```python
from build123d import *

# Parameters (mm, degrees)
SKETCH_R        = 35
SKETCH_R_2      = 32.5
PAD_DEPTH       = 2
SKETCH001_R     = 51
SKETCH001_R_2   = 32.5
PAD001_DEPTH    = 3
SKETCH002_R     = 41
SKETCH002_R_2   = 37.5
PAD002_DEPTH    = 10
SKETCH003_R     = 1.6
POCKET_DEPTH    = 5.001
CHAMFER_SIZE    = 0.5
CHAMFER001_SIZE = 1


with BuildPart() as part:
    # Sketch → Pad (new body)
    with BuildSketch(Plane.XY):
        Circle(SKETCH_R)
        Circle(SKETCH_R_2, mode=Mode.SUBTRACT)
    extrude(amount=PAD_DEPTH)

    # Sketch001 (on Face4 of Pad) → Pad001 (join)
    with BuildSketch(Plane.XY.offset(2)):
        Circle(SKETCH001_R)
        Circle(SKETCH001_R_2, mode=Mode.SUBTRACT)
    extrude(amount=PAD001_DEPTH)

    # Sketch002 (on Face7 of Pad001) → Pad002 (join)
    with BuildSketch(Plane.XY.offset(5)):
        Circle(SKETCH002_R)
        Circle(SKETCH002_R_2, mode=Mode.SUBTRACT)
    extrude(amount=PAD002_DEPTH)

    # Sketch003 (on Face7 of Pad002) → Pocket (cut, through all)
    with BuildSketch(Plane.XY.offset(5)):
        with Locations((-23, 39.837169)):
            Circle(SKETCH003_R)
        with Locations((23, 39.837169)):
            Circle(SKETCH003_R)
        with Locations((46, 0)):
            Circle(SKETCH003_R)
        with Locations((23, -39.837169)):
            Circle(SKETCH003_R)
        with Locations((-23, -39.837169)):
            Circle(SKETCH003_R)
        with Locations((-46, 0)):
            Circle(SKETCH003_R)
    extrude(amount=-POCKET_DEPTH, mode=Mode.SUBTRACT)

    # Chamfer
    chamfer_edges = [part.edges().sort_by_distance(p)[0] for p in [
        (-35, 0, 0),
    ]]
    chamfer(chamfer_edges, length=CHAMFER_SIZE)

    # Chamfer001
    chamfer001_edges = [part.edges().sort_by_distance(p)[0] for p in [
        (-37.5, 0, 15),
    ]]
    chamfer(chamfer001_edges, length=CHAMFER001_SIZE)


solid = part.part
```
For this review, take the finished solid that the model builds, in its own axes (mm). A direction names the side the tool comes from. Give positions to 0.01 mm unless a question says otherwise; leave off trailing zeros. Write each loop counter-clockwise with the first axis right and the second up, starting at its lowest first coordinate (ties: lowest second). Pieces come first, ordered by that corner, then holes.
Item 1: The part is to be moulded in two halves that separate along X. For faces 1 (the face through (-22.9, 34.2, 5)), 2 (the face through (22.792, 41.424, 3.521)), 3 (the face through (-11.056, -49.787, 3.479)), say which applies: +X half, -X half, draft (parallel to the pull), parting line (faces both ways), or undercut.
Item 2: Insertion check: P1, Ø3.5, axis at x = 46, y = 0, coming from the -Z side; P2, Ø10, axis at x = 38, y = -28, coming from the +Z side; P3, Ø3, axis at x = -7, z = 9, coming from the +Y side. Each pin has a flat end and moves straight along its axis. Give the tip position at first contact, or say it passes through.
Item 3: Machinability: for faces 4 (the face through (-4.88, 37.18, 9.44)), 5 (the face through (-47.18, 1.08, 3.52)), 6 (the face through (-28, -21, 1)), which of the approach directions +Z, -Z, +X, -X, +Y, -Y give a long, thin tool a straight path to every point of the face, cutting with its end or side? Answer none if there is none.
Item 4: Take a section at C-C (z = 12.25). Give the boundary of the cut face in (x, y), and give its area (3 significant figures).
Item 5: Take a section at A-A (y = 0). Give the number of separate pieces and of enclosed holes in the cut face, and give its area (3 significant figures).
Item 6: Take a section at B-B (x = 0). Give the boundary of the cut face in (y, z), and give its area (3 significant figures).
Item 7: Wall thickness on probe 1 along Y at (x, z) = (0, 2.45); probe 2 along Z at (x, y) = (-30.5, 38); probe 3 along Y at (x, z) = (0, 12): over which ranges is each line inside the solid? List them lowest first.
Established:
1. face 1: draft
1. face 2: undercut
1. face 3: parting line
2. P1: stops at z = 2
2. P2: stops at z = 5
2. P3: stops at y = 40.63
3. face 4: +Z
3. face 5: +Z, -Z
3. face 6: -Z
4. outline: circle Ø82 at (0, 0); hole circle Ø75 at (0, 0)
4. area: 863 mm2
5. separate pieces: 4
5. enclosed holes: 0
5. area: 171 mm2
6. outline: (-51, 2) - (-35, 2) - (-35, 0.5) - (-34.5, 0) - (-32.5, 0) - (-32.5, 5) - (-37.5, 5) - (-37.5, 14) - (-38.5, 15) - (-41, 15) - (-41, 5) - (-51, 5) - close; (32.5, 0) - (34.5, 0) - (35, 0.5) - (35, 2) - (51, 2) - (51, 5) - (41, 5) - (41, 15) - (38.5, 15) - (37.5, 14) - (37.5, 5) - (32.5, 5) - close
6. area: 190 mm2
7. probe 1: y = -51 to -32.5, 32.5 to 51
7. probe 2: z = 2 to 5
7. probe 3: y = -41 to -37.5, 37.5 to 41
